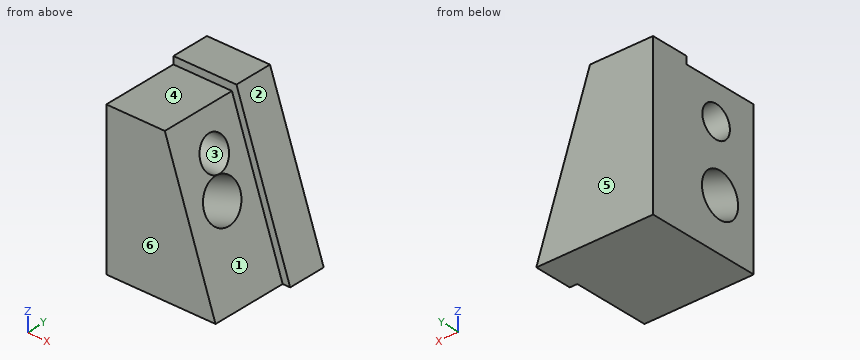
```python
from build123d import *

# Parameters (mm, degrees)
F1_DEPTH      = 76.2
F2_DEPTH      = 25.4
F3_R          = 13.6695760471
F4_DEPTH      = 120.65
F5_R          = 10.4216060464
F6_DEPTH      = 108.204
F6_DEPTH_BACK = 97.028


with BuildPart() as f1:
    # F0 (on Front) → F1 (new body)
    with BuildSketch(Plane.XZ):
        Polygon((36.0692664981, -49.5205111802), (2.5906101801, 49.5205111802), (-36.0692664981, 49.5205111802), (-36.0692664981, -49.5205111802), align=None)
    extrude(amount=F1_DEPTH)

    # F0 (on Front) → F2 (join)
    with BuildSketch(Plane.XZ):
        Polygon((36.0692664981, -49.5205111802), (2.5906101801, 49.5205111802), (-36.0692664981, 49.5205111802), (-36.0692664981, -49.5205111802), align=None)
        Polygon((-36.0692664981, 49.5205111802), (2.5906101801, 49.5205111802), (36.0692664981, -49.5205111802), (41.0287082195, -49.5205111802), (5.5572725832, 54.4315949082), (-36.0692664981, 54.4315949082), align=None)
    extrude(amount=F2_DEPTH)

    # F3 (on face) → F4 (cut)
    with BuildSketch(Plane(origin=(17.3477334247, 0, 5.8640227189), x_dir=(0, 1, 0), z_dir=(0.9473405682, 0, 0.3202278061))):
        with Locations((-50.689227879, -2.7265385725)):
            Circle(F3_R)
    extrude(amount=-F4_DEPTH, mode=Mode.SUBTRACT)

    # F5 (on Right) → F6 (cut, two sides)
    with BuildSketch(Plane.YZ) as f6_sk:
        with Locations((-47.7300770581, 26.4613311738)):
            Circle(F5_R)
    extrude(amount=F6_DEPTH, mode=Mode.SUBTRACT)
    extrude(f6_sk.sketch, amount=-F6_DEPTH_BACK, mode=Mode.SUBTRACT)


solid = f1.part
```
Part model, mm, in its own coordinate system. Face numbers are marked on the shaded views. A direction names the side the tool comes from. Round coordinates to 2 decimals unless told otherwise and drop trailing zeros. Order: outer loops, then holes, each group sorted by start corner. A loop starts at its lowest first (then second) coordinate and runs counter-clockwise, first axis right, second up. Notation, with made-up numbers: M -14,-3.75 L 11,-3.75 A27 ccw 11,29.25 Z; hole C -36.5,87.5 d5. An arc over 180 degrees is marked long. Answer in a Markdown table with one row per item. Add a question column.
Q1. Pin check, flat tip, straight feed: pin 1 (4 mm diameter, centred on y = -21, z = -9, fed in from +X). Stop position of the tip, or through.
Q2. Cut at C-C on y = -61.5. Give the cut face in (x, z).
Q3. Cut at A-A on y = -41. Give the cut face in (x, z) (3 decimals).
Q4. Mould opens along Y. For the marked faces 3, 4, 5 and 6 say: +Y half, -Y half, draft (parallel to the pull), parting line (faces both ways), or undercut.
Q5. Cut at D-D on x = 33. Give the cut face in (y, z).
Q6. Cut at B-B on z = 34.5. Give the cut face in (x, y).
Q7. 3-axis set-ups, long thin cutter, end or side, ignore diameter. For the marked faces 1 and 2: which of +Z, -Z, +X, -X, +Y, -Y reach the whole face in a straight line?
Q8. Wall check: L1, parallel to Z at x = -16.5, y = -39; L2, parallel to Y at x = 3, z = 36; L3, parallel to Z at x = 9.5, y = -39.5. Give the ranges that are in metal, low to high. Write a range as from..to.
Established:
| question | item | result |
|---|---|---|
| 1 | pin 1 | stops at x = 27.88 |
| 2 | outline | M -36.07,-49.52 L 36.07,-49.52 L 20.9,-4.64 L -36.07,-23.9 Z; M -36.07,-6.24 L 15.54,11.21 L 2.59,49.52 L -36.07,49.52 Z |
| 3 | outline | M -36.069,-49.521 L 36.069,-49.521 L 21.309,-5.854 L -36.069,-25.249 Z; M -36.069,-4.892 L 15.133,12.416 L 13.075,18.504 L -36.069,18.504 Z; M -36.069,34.418 L 7.696,34.418 L 2.591,49.521 L -36.069,49.521 Z |
| 4 | face 3 | undercut |
| 4 | face 4 | draft |
| 4 | face 5 | +Y half |
| 4 | face 6 | -Y half |
| 5 | outline | M -76.2,-49.52 L 0,-49.52 L 0,-25.99 L -25.4,-25.99 L -25.4,-40.44 L -76.2,-40.44 Z |
| 6 | outline | M -36.07,-76.2 L 7.67,-76.2 L 7.67,-54.36 L -36.07,-54.36 Z; M -36.07,-41.1 L 7.67,-41.1 L 7.67,-25.4 L 12.36,-25.4 L 12.36,0 L -36.07,0 Z |
| 7 | face 1 | +Z, +X, -Y |
| 7 | face 2 | +Z, +X, +Y, -Y |
| 8 | L1 | z = -49.52..-15.94, -0.98..20.77, 32.15..49.52 |
| 8 | L2 | y = -76.2..-51.93, -43.53..0 |
| 8 | L3 | z = -49.52..-7.96, 8.62..20.07 |
